Input: dimensioned drawing with shaded views. Units: mm. Origin: part minimum x, y, z. Give positions to 0.01 mm unless a question says otherwise; leave off trailing zeros. Write each loop counter-clockwise with the first axis right and the second up, starting at its lowest first coordinate (ties: lowest second). Pieces come first, ordered by that corner, then holes. Notation, with made-up numbers: (21.5, 55) -> (40.5, 55) arc R23 cw to (40.5, 85) -> close; hole circle Ø4 at (30.25, -39). An arc over 180 degrees is marked (long way). Return JSON: item names as keys, results as strings. Group by question number.
Item 1: Line query: line 1 (X direction, y = 2.85, z = 18); line 2 (X direction, y = 0.5, z = 29). Output: solid intervals per line, ascending. Write a range as [from, to].
Item 2: Pin query (flat end, axial travel): P1, Ø1, axis at y = 1.5, z = 8.5, coming from the +X side; P2, Ø1, axis at y = 2, z = 10.5, coming from the -X side. Return the tip coordinate at first contact, or that it passes through.
Item 3: Section A-A, the plane y = 0.8. Return loops of the section in (x, z), then the cut area to 3 significant figures.
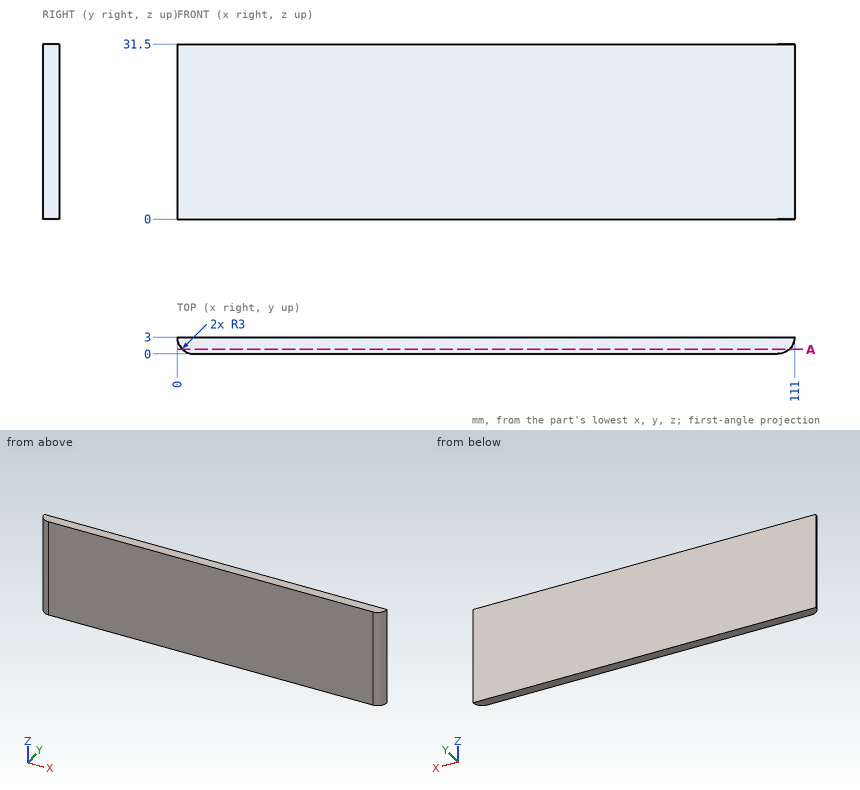
Answer below:
{
 "1": {"line 1": "x = [0, 111]", "line 2": "x = [1.34, 109.66]"},
 "2": {"P1": "stops at x = 110.83", "P2": "stops at x = 0.04"},
 "3": {"outline": "(0.96, 0) -> (110.04, 0) -> (110.04, 31.5) -> (0.96, 31.5) -> close", "area": "3,440 mm2"}
}
